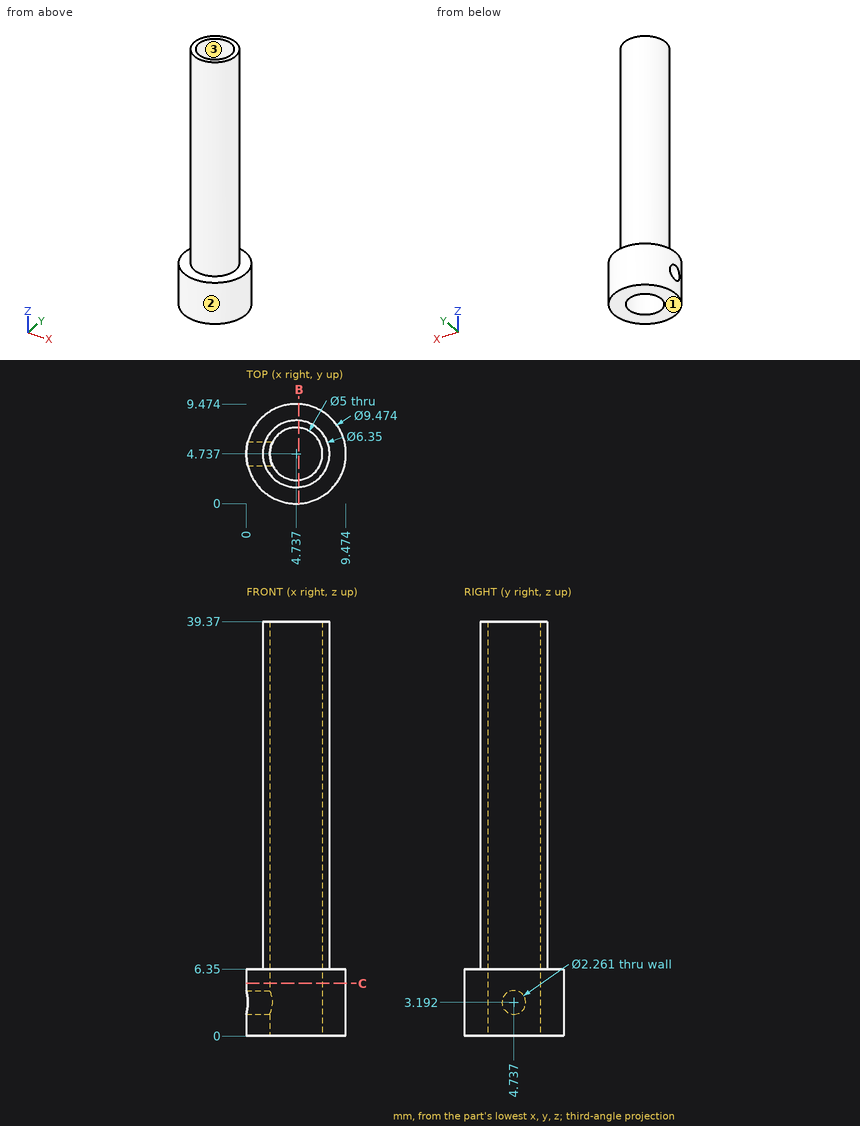
Answer from the drawing. Dimensions are ordinates in mm from the lowest x, y and z of the part. Round coordinates to 2 decimals unless told otherwise and drop trailing zeros. Write each loop counter-clockwise with the first axis right and the second up, starting at its lowest first coordinate (ties: lowest second). Pieces come first, ordered by that corner, then holes. Notation, with made-up numbers: (16, 14) -> (61, 14) arc R20 cw to (61, 27) -> close; hole circle Ø1 at (86.5, 71.5). An arc over 180 degrees is marked (long way). Answer in a Markdown table with one row per item. Add a question column.
1) Find section B-B, the plane x = 5. Determine the outline of the cut face in (y, z).
2) Given P1, Ø1, axis at x = 8.5, z = 22.5, coming from the +Y side; P2, Ø1.5, axis at y = 5, z = 28, coming from the +X side; P3, Ø3, axis at x = 2, z = 35, coming from the -Y side; P4, Ø2, axis at x = 8.5, z = 15, coming from the -Y side (1 decimal), each flat-ended and moving along its own axis, determine where each tip first touches the part or whether it passes through.
3) Consider line 1 (X direction, y = 3.25, z = 6) (1 decimal); line 2 (Z direction, x = 1, y = 3.5); line 3 (X direction, y = 5, z = 14). Determine where each line is inside the solid, lowest interval first.
4) Find section C-C, the plane z = 5. Determine the outline of the cut face in (x, y) (1 decimal).
5) Determine the mould class of the marked faces 1, 2 and 3 for opening direction X: pulls with the +X half, pulls with the -X half, needs draft (parallel to the pull), parting line crosses it, or undercut.
Findings below:
| question | item | result |
|---|---|---|
| 1 | outline | (0.01, 0) -> (2.25, 0) -> (2.25, 39.37) -> (1.57, 39.37) -> (1.57, 6.35) -> (0.01, 6.35) -> close; (7.22, 0) -> (9.47, 0) -> (9.47, 6.35) -> (7.9, 6.35) -> (7.9, 39.37) -> (7.22, 39.37) -> close |
| 2 | P1 | through |
| 2 | P2 | x = 7.91 |
| 2 | P3 | y = 1.81 |
| 2 | P4 | y = 3.2 |
| 3 | line 1 | 0.2 to 2.7, 6.7 to 9.2 |
| 3 | line 2 | 0 to 6.35 |
| 3 | line 3 | 1.57 to 2.25, 7.22 to 7.9 |
| 4 | outline | circle Ø9.5 at (4.7, 4.7); hole circle Ø5 at (4.7, 4.7) |
| 5 | face 1 | needs draft |
| 5 | face 2 | parting line crosses it |
| 5 | face 3 | undercut |
